For this review, take the finished solid that the model builds, in its own axes (mm). Face numbers are marked on the shaded views. Round coordinates to 2 decimals unless told otherwise and drop trailing zeros. Order: outer loops, then holes, each group sorted by start corner. A loop starts at its lowest first (then second) coordinate and runs counter-clockwise, first axis right, second up. Notation, with made-up numbers: (-36, 24) - (-26, 24) arc R10 cw to (-26, 40) - close; hole circle Ø7 at (22, 68). An arc over 180 degrees is marked (long way). One line per question, with ' | ' between items.
```python
from build123d import *

# Parameters (mm, degrees)
SKETCH1_W           = 70
SKETCH1_H           = 70
BOSS_EXTRUDE1_DEPTH = 2.5
FILLET1_R           = 8
CUT_EXTRUDE1_DEPTH  = 2.75
SKETCH3_R           = 2.25
BOSS_EXTRUDE2_DEPTH = 2.75
CHAMFER1_SIZE       = 0.15


with BuildPart() as part:
    # Sketch1 → Boss-Extrude1 (new body, symmetric)
    with BuildSketch(Plane(origin=(0, 0, 0), x_dir=(1, 0, 0), z_dir=(0, 1, 0))):
        Rectangle(SKETCH1_W, SKETCH1_H)
    extrude(amount=BOSS_EXTRUDE1_DEPTH, both=True)

    # Fillet1
    fillet1_edges = [part.edges().sort_by_distance(p)[0] for p in [
        (35, 0, 35),
        (-35, 0, 35),
        (-35, 0, -35),
        (35, 0, -35),
    ]]
    fillet(fillet1_edges, radius=FILLET1_R)

    # Sketch2 → Cut-Extrude1 (cut)
    with BuildSketch(Plane(origin=(0, 2.5, 0), x_dir=(1, 0, 0), z_dir=(0, 1, 0))):
        with BuildLine():
            Line((32.75, -27), (32.75, 27))
            ThreePointArc((32.75, 27), (31.065863992, 31.065863992), (27, 32.75))
            Line((27, 32.75), (-27, 32.75))
            ThreePointArc((-27, 32.75), (-31.065863992, 31.065863992), (-32.75, 27))
            Line((-32.75, 27), (-32.75, -27))
            ThreePointArc((-32.75, -27), (-31.065863992, -31.065863992), (-27, -32.75))
            Line((-27, -32.75), (27, -32.75))
            ThreePointArc((27, -32.75), (31.065863992, -31.065863992), (32.75, -27))
        make_face()
    extrude(amount=-CUT_EXTRUDE1_DEPTH, mode=Mode.SUBTRACT)

    # Sketch3 → Boss-Extrude2 (add)
    with BuildSketch(Plane(origin=(0, -0.25, 0), x_dir=(1, 0, 0), z_dir=(0, 1, 0))):
        with Locations((-20, 20)):
            Circle(SKETCH3_R)
        with Locations((0, 20)):
            Circle(SKETCH3_R)
        with Locations((20, 20)):
            Circle(SKETCH3_R)
        Circle(SKETCH3_R)
        with Locations((20, 0)):
            Circle(SKETCH3_R)
        with Locations((0, -20)):
            Circle(SKETCH3_R)
        with Locations((20, -20)):
            Circle(SKETCH3_R)
        with Locations((-20, 0)):
            Circle(SKETCH3_R)
        with Locations((-20, -20)):
            Circle(SKETCH3_R)
    extrude(amount=BOSS_EXTRUDE2_DEPTH)

    # Chamfer1
    chamfer1_edges = [part.edges().sort_by_distance(p)[0] for p in [
        (35, 2.5, 0),
        (35, -2.5, 0),
        (0, 2.5, -35),
        (-35, 2.5, 0),
        (0, 2.5, 35),
        (-32.656854249, 2.5, 32.656854249),
        (-32.656854249, 2.5, -32.656854249),
        (32.656854249, 2.5, 32.656854249),
        (32.656854249, 2.5, -32.656854249),
        (0, -2.5, -35),
        (0, -2.5, 35),
        (-35, -2.5, 0),
        (-32.656854249, -2.5, 32.656854249),
        (-32.656854249, -2.5, -32.656854249),
        (32.656854249, -2.5, 32.656854249),
        (32.656854249, -2.5, -32.656854249),
        (31.065863992, 2.5, -31.065863992),
        (0, 2.5, -32.75),
        (-31.065863992, 2.5, -31.065863992),
        (-32.75, 2.5, 0),
        (-31.065863992, 2.5, 31.065863992),
        (0, 2.5, 32.75),
        (31.065863992, 2.5, 31.065863992),
        (32.75, 2.5, 0),
        (-22.25, 2.5, -20),
        (-2.25, 2.5, -20),
        (17.75, 2.5, -20),
        (-2.25, 2.5, 0),
        (17.75, 2.5, 0),
        (-2.25, 2.5, 20),
        (17.75, 2.5, 20),
        (-22.25, 2.5, 0),
        (-22.25, 2.5, 20),
    ]]
    chamfer(chamfer1_edges, length=CHAMFER1_SIZE)


solid = part.part
```
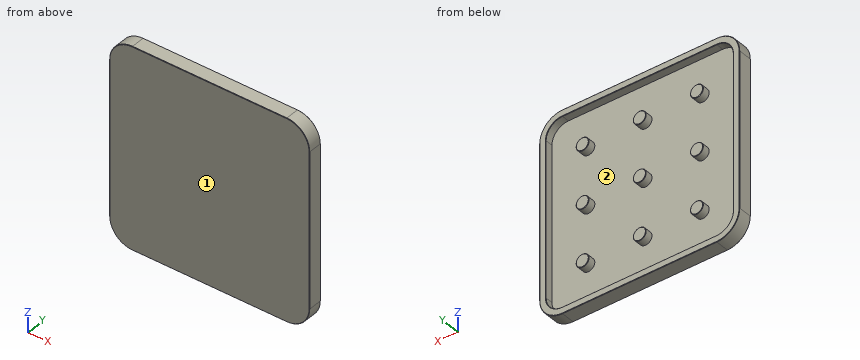
(1) We need section C-C on x = 5.5. State the section outline as (y, z) points.
Output values:
outline: (-2.5, -34.85) - (-2.35, -35) - (2.35, -35) - (2.5, -34.85) - (2.5, -32.9) - (2.35, -32.75) - (-0.25, -32.75) - (-0.25, 32.75) - (2.35, 32.75) - (2.5, 32.9) - (2.5, 34.85) - (2.35, 35) - (-2.35, 35) - (-2.5, 34.85) - close
(2) Mouldability with a two-part tool opening along Z and no side actions: class the marked faces 1 and 2 as released by +Z, released by -Z, zero draft, split by the parting line, or undercut.
Output values:
face 1: zero draft | face 2: undercut
(3) Insertion check: pin 1 (2 mm diameter, centred on x = 14.5, z = -2.5, fed in from +Y). The pin has a flat end and moves straight along its axis. Give the tip position at first contact, or say it passes through.
Output values:
pin 1: y = -0.25
(4) For probe 1 along X at (y, z) = (0.1, -7.5); probe 2 along X at (y, z) = (0.55, 18.5), list the stretches that pass through material, from the lowest coordinate up. Write a range as [from, to].
Output values:
probe 1: [-35, -32.75], [32.75, 35] | probe 2: [-35, -32.75], [-21.68, -18.32], [-1.68, 1.68], [18.32, 21.68], [32.75, 35]
